The listing builds one solid part. Answer for the finished solid, in the listing's coordinates (mm). A direction names the side the tool comes from. Coordinates: 2 decimals unless noted, no trailing zeros. Write each loop counter-clockwise with the first axis right and the second up, starting at its lowest first coordinate (ties: lowest second). Pieces come first, ordered by that corner, then holes.
(1) The part is cut by section B-B on y = 3.75. Give the number of separate pieces and of enclosed holes in the cut face, plus the area to 3 significant figures.
(2) The part is cut by section A-A on z = 0. Determine the outline of the cut face in (x, y).
(3) Which of the six approach directions +Z, -Z, +X, -X, +Y, -Y give full straight-line access (tool end or side, diameter ignored) to faces 4 (the flat face through (103, 3, -79.375)), 5 (the flat face through (60.673, 3, 1)), 6 (the flat face through (-104, 3, -79.375)), 7 (the flat face through (104, 3, 79.375)), 8 (the flat face through (-103, 3, 79.375))?
(4) Given P1, Ø1.5, axis at x = 96, y = 3, coming from the -Z side (3 decimals); P2, Ø1.9, axis at x = -93, y = 3.5, coming from the +Z side (3 decimals); P3, Ø2.5, axis at y = 3.5, z = -81, coming from the -X side, each flat-ended and moving along its own axis, determine where each tip first touches the part or whether it passes through.
(5) For a pull along Z with two mould halves and no side action, classify faces 1 (the flat face through (-1, 3, 82.55)), 2 (the flat face through (146.05, 3, -1)), 3 (the flat face through (-25.4, 3, 0)) as +Z half, -Z half, draft (parallel to the pull), parting line (faces both ways), or undercut.
(6) Straight lines are drawn through the part: line 1 (Z direction, x = -30, y = 5.75); line 2 (X direction, y = 6, z = -16); line 3 (X direction, y = 4.25, z = -51). For each, find the intervals that lie inside material, in ascending order.
from build123d import *

# Parameters (mm, degrees)
BOSS_EXTRUDE1_DEPTH     = 6.35
SKETCH2_W               = 25.4
SKETCH2_H               = 12.7
CUT_EXTRUDE1_DEPTH      = 186.567817792
SKETCH6_W               = 203.2
SKETCH6_H               = 34.925
CUT_EXTRUDE3_DEPTH      = 186.567817792
SKETCH9_W               = 127
SKETCH9_H               = 3.175
BOSS_EXTRUDE3_DEPTH     = 6.35
SKETCH12_R              = 1.5875
CUT_EXTRUDE5_DEPTH      = 168.885161643
MIRROR2_COPY_1_SKETCH_R = 1.5875
MIRROR2_COPY_1_DEPTH    = 168.885161643
SKETCH13_R              = 25
CUT_EXTRUDE6_DEPTH      = 168.885161643
SKETCH15_W              = 33.02
SKETCH15_H              = 106
CUT_EXTRUDE7_DEPTH      = 168.885161643


with BuildPart() as part:
    # Sketch1 → Boss-Extrude1 (new body)
    with BuildSketch(Plane.XZ):
        with BuildLine():
            Line((142.875, 79.375), (66.817002043, 79.375))
            ThreePointArc((66.817002043, 79.375), (64.571938013, 80.30493597), (63.642002043, 82.55))
            Line((63.642002043, 82.55), (63.642002043, 111.125))
            ThreePointArc((63.642002043, 111.125), (62.712066074, 113.37006403), (60.467002043, 114.3))
            Line((60.467002043, 114.3), (-60.467002043, 114.3))
            ThreePointArc((-60.467002043, 114.3), (-62.712066074, 113.37006403), (-63.642002043, 111.125))
            Line((-63.642002043, 111.125), (-63.642002043, 82.55))
            ThreePointArc((-63.642002043, 82.55), (-64.571938013, 80.30493597), (-66.817002043, 79.375))
            Line((-66.817002043, 79.375), (-142.875, 79.375))
            ThreePointArc((-142.875, 79.375), (-145.12006403, 78.44506403), (-146.05, 76.2))
            Line((-146.05, 76.2), (-146.05, -76.2))
            ThreePointArc((-146.05, -76.2), (-145.12006403, -78.44506403), (-142.875, -79.375))
            Line((-142.875, -79.375), (-66.817002043, -79.375))
            ThreePointArc((-66.817002043, -79.375), (-64.571938013, -80.30493597), (-63.642002043, -82.55))
            Line((-63.642002043, -82.55), (-63.642002043, -111.125))
            ThreePointArc((-63.642002043, -111.125), (-62.712066074, -113.37006403), (-60.467002043, -114.3))
            Line((-60.467002043, -114.3), (60.467002043, -114.3))
            ThreePointArc((60.467002043, -114.3), (62.712066074, -113.37006403), (63.642002043, -111.125))
            Line((63.642002043, -111.125), (63.642002043, -82.55))
            ThreePointArc((63.642002043, -82.55), (64.571938013, -80.30493597), (66.817002043, -79.375))
            Line((66.817002043, -79.375), (142.875, -79.375))
            ThreePointArc((142.875, -79.375), (145.12006403, -78.44506403), (146.05, -76.2))
            Line((146.05, -76.2), (146.05, 76.2))
            ThreePointArc((146.05, 76.2), (145.12006403, 78.44506403), (142.875, 79.375))
        make_face()
    extrude(amount=-BOSS_EXTRUDE1_DEPTH)

    # Sketch2 → Cut-Extrude1 (cut, through all)
    with BuildSketch(Plane(origin=(0, 6.35, 0), x_dir=(1, 0, 0), z_dir=(0, 1, 0))):
        with Locations((-38.1, 0)):
            Rectangle(SKETCH2_W, SKETCH2_H)
    extrude(amount=-CUT_EXTRUDE1_DEPTH, mode=Mode.SUBTRACT)

    # Sketch6 → Cut-Extrude3 (cut, through all)
    with BuildSketch(Plane.XZ):
        with Locations((0, 96.8375)):
            Rectangle(SKETCH6_W, SKETCH6_H)
        with Locations((0, -96.8375)):
            Rectangle(SKETCH6_W, SKETCH6_H)
    extrude(amount=-CUT_EXTRUDE3_DEPTH, mode=Mode.SUBTRACT)

    # Sketch9 → Boss-Extrude3 (add)
    with BuildSketch(Plane(origin=(0, 6.35, 0), x_dir=(1, 0, 0), z_dir=(0, 1, 0))):
        with Locations((0, 80.9625)):
            Rectangle(SKETCH9_W, SKETCH9_H)
        with Locations((0, -80.9625)):
            Rectangle(SKETCH9_W, SKETCH9_H)
    extrude(amount=-BOSS_EXTRUDE3_DEPTH)

    # Sketch12 → Cut-Extrude5 (cut, symmetric)
    with BuildSketch(Plane.XZ):
        with Locations(Location((-128.905, 64.825, 0), (0, 0, 270))):
            Circle(SKETCH12_R)
        with Locations(Location((-88.265, 64.825, 0), (0, 0, 270))):
            Circle(SKETCH12_R)
        with Locations(Location((-101.289228739, 46.585, 0), (0, 0, 270))):
            Circle(SKETCH12_R)
        with Locations(Location((-101.289228739, 33.885, 0), (0, 0, 270))):
            Circle(SKETCH12_R)
        with Locations(Location((-115.880769, 33.885, 0), (0, 0, 270))):
            Circle(SKETCH12_R)
        with Locations(Location((-115.880769, 46.585, 0), (0, 0, 270))):
            Circle(SKETCH12_R)
    cut_extrude5 = extrude(amount=CUT_EXTRUDE5_DEPTH, both=True, mode=Mode.SUBTRACT)

    # Mirror1: Cut-Extrude5 across plane
    add(cut_extrude5.mirror(Plane(origin=(0, 0, 0), x_dir=(0, 0, 1), z_dir=(1, 0, 0))), mode=Mode.SUBTRACT)

    # Mirror2: Cut-Extrude5 across plane
    add(cut_extrude5.mirror(Plane(origin=(0, 0, 0), x_dir=(1, 0, 0), z_dir=(0, 0, -1))), mode=Mode.SUBTRACT)

    # Mirror2 copy 1 sketch → Mirror2 copy 1 (cut, symmetric)
    with BuildSketch(Plane(origin=(0, 0, 0), x_dir=(-1, 0, 0), z_dir=(0, -1, 0))):
        with Locations(Location((-128.905, 64.825, 0), (0, 0, 270))):
            Circle(MIRROR2_COPY_1_SKETCH_R)
        with Locations(Location((-88.265, 64.825, 0), (0, 0, 270))):
            Circle(MIRROR2_COPY_1_SKETCH_R)
        with Locations(Location((-101.289228739, 46.585, 0), (0, 0, 270))):
            Circle(MIRROR2_COPY_1_SKETCH_R)
        with Locations(Location((-101.289228739, 33.885, 0), (0, 0, 270))):
            Circle(MIRROR2_COPY_1_SKETCH_R)
        with Locations(Location((-115.880769, 33.885, 0), (0, 0, 270))):
            Circle(MIRROR2_COPY_1_SKETCH_R)
        with Locations(Location((-115.880769, 46.585, 0), (0, 0, 270))):
            Circle(MIRROR2_COPY_1_SKETCH_R)
    extrude(amount=MIRROR2_COPY_1_DEPTH, both=True, mode=Mode.SUBTRACT)

    # Sketch13 → Cut-Extrude6 (cut, through all)
    with BuildSketch(Plane(origin=(0, 6.35, 0), x_dir=(1, 0, 0), z_dir=(0, 1, 0))):
        with Locations(Location((88.21149281, 0, 0), (0, 0, 270))):
            Circle(SKETCH13_R)
    extrude(amount=-CUT_EXTRUDE6_DEPTH, mode=Mode.SUBTRACT)

    # Sketch15 → Cut-Extrude7 (cut, through all)
    with BuildSketch(Plane(origin=(0, 6.35, 0), x_dir=(1, 0, 0), z_dir=(0, 1, 0))):
        with Locations((44.163037407, 0)):
            Rectangle(SKETCH15_W, SKETCH15_H)
    extrude(amount=-CUT_EXTRUDE7_DEPTH, mode=Mode.SUBTRACT)


solid = part.part
Model answer:
1. separate pieces: 1
1. enclosed holes: 27
1. area: 41,200 mm2
2. outline: (-146.05, 0) - (-50.8, 0) - (-50.8, 6.35) - (-146.05, 6.35) - close; (-25.4, 0) - (27.65, 0) - (27.65, 6.35) - (-25.4, 6.35) - close; (60.67, 0) - (63.21, 0) - (63.21, 6.35) - (60.67, 6.35) - close; (113.21, 0) - (146.05, 0) - (146.05, 6.35) - (113.21, 6.35) - close
3. face 4: -Z, +X, +Y, -Y
3. face 5: +Y, -Y
3. face 6: -Z, -X, +Y, -Y
3. face 7: +Z, +X, +Y, -Y
3. face 8: +Z, -X, +Y, -Y
4. P1: stops at z = -79.375
4. P2: stops at z = 79.375
4. P3: stops at x = -63.5
5. face 1: +Z half
5. face 2: draft
5. face 3: undercut
6. line 1: z = -82.55 to -6.35, 6.35 to 82.55
6. line 2: x = -146.05 to 27.65, 60.67 to 69, 107.42 to 146.05
6. line 3: x = -146.05 to 27.65, 60.67 to 146.05
